Source: three-view drawing plus pictorial views. Frame: mm from the lowest corner of the part. A direction names the side the tool comes from. Give positions to 0.01 mm unless a question says otherwise; leave off trailing zeros. Loops run counter-clockwise (first coordinate to the right, second up) from the corner with the lowest first, then second, coordinate; pieces in that order, holes last. Notation, with made-up numbers: M 30,18.5 L 50,18.5 A31 ccw 50,50.5 Z; hole C 44.5,32 d6. An arc over 180 degrees is marked long. Put each result on its own line as item: value. Start each with the question number.
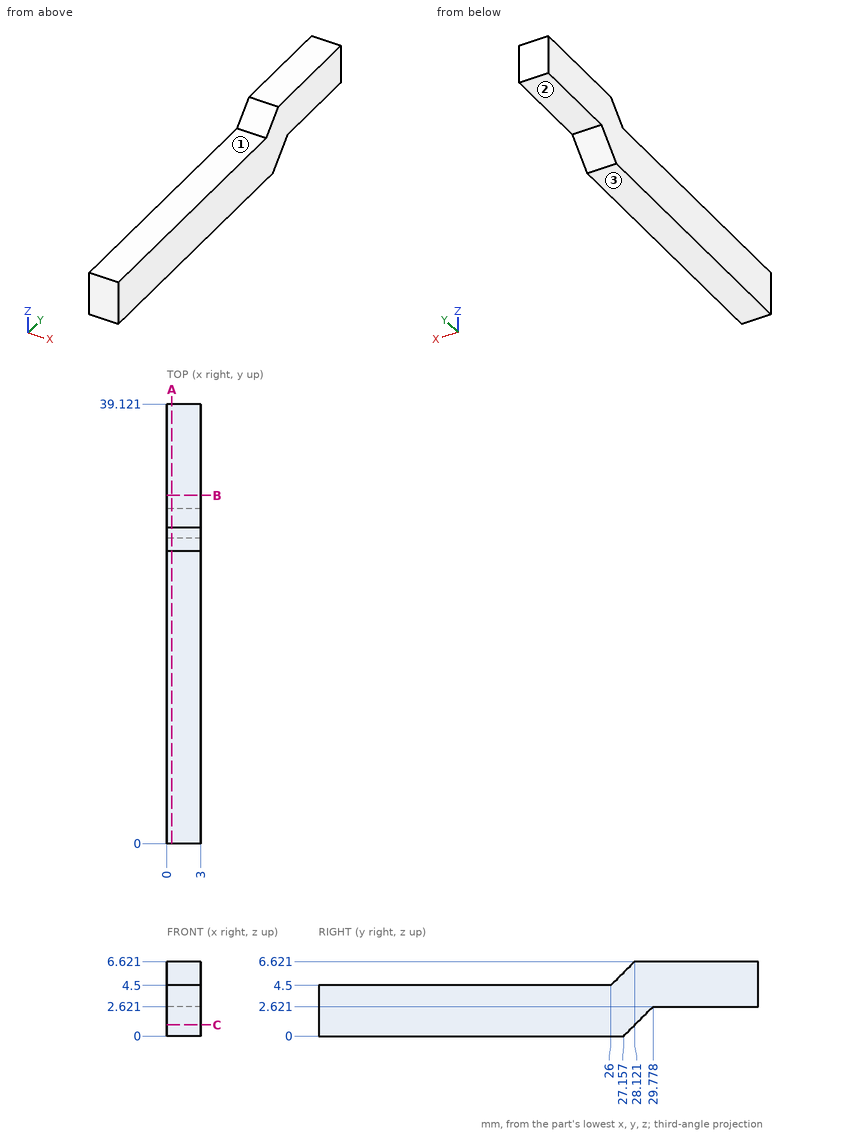
1. Section B-B, the plane y = 31. Output: boundary loops of the cut face in (x, z).
2. Section C-C, the plane z = 1. Output: boundary loops of the cut face in (x, y).
3. Ray query, line 1 (Z direction, x = 0.65, y = 7); line 2 (Z direction, x = 2.4, y = 36); line 3 (Y direction, x = 0.2, z = 1.25) (1 decimal). Return the intervals inside material, ascending.
4. Section A-A, the plane x = 0.45. Output: boundary loops of the cut face in (y, z), plus the area to 3 significant figures.
5. Set-up query: the marked faces 1, 2 and 3. Return all of +Z, -Z, +X, -X, +Y, -Y with unobstructed straight access to the full face (end or side cutting, diameter ignored); none if empty.
6. Contact query for flat-ended pins moving along their axis: pin 1 (1.5 mm diameter, centred on x = 2, y = 8.5, fed in from +Z); pin 2 (0.9 mm diameter, centred on x = 1, y = 34, fed in from -Z). Output: stop coordinate, or through.
Results found:
1. outline: M 0,2.62 L 3,2.62 L 3,6.62 L 0,6.62 Z
2. outline: M 0,0 L 3,0 L 3,28.16 L 0,28.16 Z
3. line 1: 0 to 4.5
3. line 2: 2.62 to 6.62
3. line 3: 0 to 28.4
4. outline: M 0,0 L 27.16,0 L 29.78,2.62 L 39.12,2.62 L 39.12,6.62 L 28.12,6.62 L 26,4.5 L 0,4.5 Z
4. area: 174 mm²
5. face 1: +Z, +X, -X, -Y
5. face 2: -Z, +X, -X, +Y
5. face 3: -Z, +X, -X, +Y, -Y
6. pin 1: z = 4.5
6. pin 2: z = 2.62
